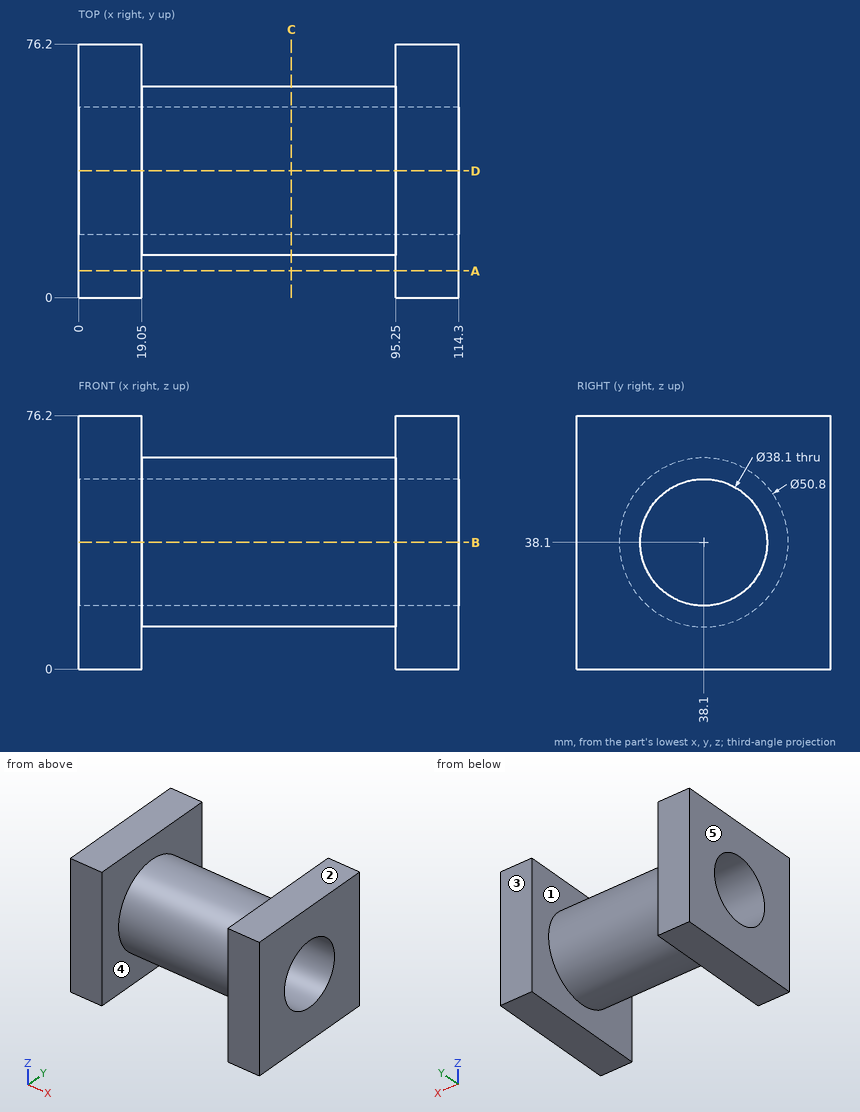
Drawing for the job (mm, zero at the part's lowest x, y, z). A direction names the side the tool comes from. Round coordinates to 2 decimals unless told otherwise and drop trailing zeros. Order: outer loops, then holes, each group sorted by start corner. A loop starts at its lowest first (then second) coordinate and runs counter-clockwise, first axis right, second up.
Item 1: Tool access for the marked faces 1 and 2: list every direction of +Z, -Z, +X, -X, +Y, -Y with a clear straight run to the whole face (end or side of a thin tool).
Item 2: Saw through at B-B on z = 38.1. Write the cut outline in (x, y).
Item 3: Pin check, flat tips, straight feed: pin 1 (12 mm diameter, centred on x = 41, z = 41, fed in from +Y); pin 2 (8 mm diameter, centred on x = 88.5, y = 40, fed in from -Z); pin 3 (8 mm diameter, centred on x = 37.5, y = 26.5, fed in from -Z). Stop position of each tip, or through.
Item 4: Saw through at C-C on x = 64. Write the cut outline in (y, z).
Item 5: Probe line 1 along Z through (x, y) = (25, 38.1); line 2 along X through (y, z) = (64.5, 29.5). List the from-to ranges inside material, lowest first.
Item 6: Saw through at A-A on y = 8. Write the cut outline in (x, z), then the cut area to 3 significant figures.
Item 7: Mould opens along X. For the marked faces 3, 4 and 5 say: pulls with the +X half, pulls with the -X half, needs draft (parallel to the pull), parting line crosses it, or undercut.
Reported:
1. face 1: none
1. face 2: +Z, +X, -X, +Y, -Y
2. outline: (0, 0) - (19.05, 0) - (19.05, 12.7) - (95.25, 12.7) - (95.25, 0) - (114.3, 0) - (114.3, 19.05) - (0, 19.05) - close; (0, 57.15) - (114.3, 57.15) - (114.3, 76.2) - (95.25, 76.2) - (95.25, 63.5) - (19.05, 63.5) - (19.05, 76.2) - (0, 76.2) - close
3. pin 1: stops at y = 63.5
3. pin 2: stops at z = 12.7
3. pin 3: stops at z = 13.86
4. outline: circle Ø50.8 at (38.1, 38.1); hole circle Ø38.1 at (38.1, 38.1)
5. line 1: z = 12.7 to 19.05, 57.15 to 63.5
5. line 2: x = 0 to 19.05, 95.25 to 114.3
6. outline: (0, 0) - (19.05, 0) - (19.05, 76.2) - (0, 76.2) - close; (95.25, 0) - (114.3, 0) - (114.3, 76.2) - (95.25, 76.2) - close
6. area: 2,900 mm2
7. face 3: needs draft
7. face 4: undercut
7. face 5: pulls with the -X half
